Geometry check sheet. Reference: the model listing, model coordinates, mm. A direction names the side the tool comes from. Give positions to 0.01 mm unless a question says otherwise; leave off trailing zeros. Loops run counter-clockwise (first coordinate to the right, second up) from the corner with the lowest first, then second, coordinate; pieces in that order, holes last. Notation, with made-up numbers: (-36.5, 67.5) - (15.5, 67.5) arc R13 cw to (15.5, 82.5) - close; hole circle Ø6 at (79, 60). An arc over 180 degrees is marked (long way). One line per question, with ' | ' between items. Start each with the question number.
from build123d import *

# Parameters (mm, degrees)
SKETCH2_W           = 45.0088
SKETCH2_H           = 38.0746
SKETCH2_R           = 2.5146
BOSS_EXTRUDE1_DEPTH = 1.524
SKETCH3_W           = 10.026160074
SKETCH3_H           = 3.839196093
BOSS_EXTRUDE2_DEPTH = 29.6164
SKETCH4_R           = 18.7706
BOSS_EXTRUDE3_DEPTH = 16.51


with BuildPart() as part:
    # Sketch2 → Boss-Extrude1 (new body)
    with BuildSketch(Plane.XY):
        with Locations((22.5044, 19.0373)):
            Rectangle(SKETCH2_W, SKETCH2_H)
        with Locations(Location((4.8514, 33.2232, 0), (0, 0, 180))):
            Circle(SKETCH2_R, mode=Mode.SUBTRACT)
        with Locations(Location((4.8514, 4.8514, 0), (0, 0, 180))):
            Circle(SKETCH2_R, mode=Mode.SUBTRACT)
        with Locations(Location((40.1574, 4.8514, 0), (0, 0, 180))):
            Circle(SKETCH2_R, mode=Mode.SUBTRACT)
        with Locations(Location((40.1574, 33.2232, 0), (0, 0, 180))):
            Circle(SKETCH2_R, mode=Mode.SUBTRACT)
    extrude(amount=BOSS_EXTRUDE1_DEPTH)

    # Sketch3 → Boss-Extrude2 (add)
    with BuildSketch(Plane.XY.offset(1.524)):
        with Locations((20.750845866, 33.676355349)):
            Rectangle(SKETCH3_W, SKETCH3_H)
    extrude(amount=BOSS_EXTRUDE2_DEPTH)

    # Sketch4 → Boss-Extrude3 (add)
    with BuildSketch(Plane.XZ.offset(-31.756757303)):
        with Locations(Location((20.750845866, 31.1404, 0), (0, 0, 285.490039243))):
            Circle(SKETCH4_R)
    extrude(amount=BOSS_EXTRUDE3_DEPTH)


solid = part.part
(1) Section check C-C, the plane x = 34. Record the boundary of the cut face in (y, z).
(2) Depth check by flat-ended pin: pin 1 Ø3 at (x, y) = (40.16, 33.22) entering from +Z; pin 2 Ø3 at (x, y) = (20.5, 33.5) entering from +Z; pin 3 Ø3 at (x, z) = (7.5, 38.5) entering from +Y; pin 4 Ø3 at (x, z) = (19, 15.5) entering from +Y. Enter the tip coordinate at first touch or a pass-through.
(3) Section check D-D, the plane y = 29.5. Record the boundary of the cut face in (x, z).
(4) Tool access check on faces 5 (the face through (5.397, 35.678, 0.751)), 6 (the face through (15.738, 34, 16)), 7 (the face through (21, 35.596, 16)), 8 (the face through (25.764, 34, 16)). Record the directions out of +Z, -Z, +X, -X, +Y, -Y that give a thin tool (end or side, any length) a straight path to the whole face; none if there is none.
(5) Material ranges on line 1 (Z direction, x = 42, y = 29); line 2 (Z direction, x = 7, y = 30); line 3 (Y direction, x = 3, z = 30), recorded low to high.
(6) Section check B-B, the plane y = 34.5. Record the boundary of the cut face in (x, z), and give its area (3 significant figures).
(7) Mould release check, pull along Z, two halves, no side actions. Record for faces 1 (the face through (22, 19, 0)), 2 (the face through (18.45, 23.62, 12.51)), 3 (the face through (22, 19, 1.524)), 4 (the face through (22, 0, 1)): pulls with the +Z half, pulls with the -Z half, needs draft (parallel to the pull), parting line crosses it, or undercut.
(8) Section check A-A, the plane x = 3. Record the boundary of the cut face in (y, z), and give its area (3 significant figures).
Numbers:
1) outline: (0, 0) - (38.07, 0) - (38.07, 1.52) - (0, 1.52) - close; (15.25, 17.84) - (31.76, 17.84) - (31.76, 44.44) - (15.25, 44.44) - close
2) pin 1: through | pin 2: z = 31.14 | pin 3: y = 31.76 | pin 4: y = 35.6
3) outline: (0, 0) - (45.01, 0) - (45.01, 1.52) - (0, 1.52) - close; circle Ø37.54 at (20.75, 31.14)
4) face 5: -Z | face 6: +Z, -X, +Y | face 7: +Z, +X, -X, +Y | face 8: +Z, +X, +Y
5) line 1: 0 to 1.52 | line 2: 0 to 1.52, 18.36 to 43.92 | line 3: 15.25 to 31.76
6) outline: (0, 0) - (2.69, 0) - (2.69, 1.52) - (0, 1.52) - close; (7.02, 0) - (37.99, 0) - (37.99, 1.52) - (25.76, 1.52) - (25.76, 31.14) - (15.74, 31.14) - (15.74, 1.52) - (7.02, 1.52) - close; (42.32, 0) - (45.01, 0) - (45.01, 1.52) - (42.32, 1.52) - close | area: 352 mm^2
7) face 1: pulls with the -Z half | face 2: undercut | face 3: undercut | face 4: needs draft
8) outline: (0, 0) - (3.15, 0) - (3.15, 1.52) - (0, 1.52) - close; (6.55, 0) - (31.52, 0) - (31.52, 1.52) - (6.55, 1.52) - close; (15.25, 25.04) - (31.76, 25.04) - (31.76, 37.24) - (15.25, 37.24) - close; (34.92, 0) - (38.07, 0) - (38.07, 1.52) - (34.92, 1.52) - close | area: 249 mm^2
